from build123d import *

# Parameters (mm, degrees)
SKETCH1_W           = 94
SKETCH1_H           = 94
BOSS_EXTRUDE1_DEPTH = 11.3
SKETCH2_R           = 1.9
BOSS_EXTRUDE2_DEPTH = 2
SKETCH3_R           = 2.4
BOSS_EXTRUDE3_DEPTH = 17.9
SKETCH4_W           = 4
SKETCH4_H           = 7
CUT_EXTRUDE1_DEPTH  = 7.4


with BuildPart() as part:
    # Sketch1 → Boss-Extrude1 (new body)
    with BuildSketch(Plane(origin=(0, 0, 0), x_dir=(1, 0, 0), z_dir=(0, 1, 0))):
        with Locations((47, 47)):
            Rectangle(SKETCH1_W, SKETCH1_H)
    extrude(amount=BOSS_EXTRUDE1_DEPTH)

    # Sketch2 → Boss-Extrude2 (add)
    with BuildSketch(Plane.XZ):
        with Locations(Location((6.4, -6.4, 0), (0, 0, 270))):
            Circle(SKETCH2_R)
        with Locations(Location((6.4, -87.6, 0), (0, 0, 90))):
            Circle(SKETCH2_R)
        with Locations(Location((87.6, -87.6, 0), (0, 0, 270))):
            Circle(SKETCH2_R)
        with Locations(Location((87.6, -6.4, 0), (0, 0, 90))):
            Circle(SKETCH2_R)
    extrude(amount=BOSS_EXTRUDE2_DEPTH)

    # Sketch3 → Boss-Extrude3 (add)
    with BuildSketch(Plane(origin=(0, 11.3, 0), x_dir=(1, 0, 0), z_dir=(0, 1, 0))):
        with Locations(Location((47, 47, 0), (0, 0, 90))):
            Circle(SKETCH3_R)
    extrude(amount=BOSS_EXTRUDE3_DEPTH)

    # Sketch4 → Cut-Extrude1 (cut)
    with BuildSketch(Plane(origin=(0, 29.2, 0), x_dir=(1, 0, 0), z_dir=(0, 1, 0))):
        with Locations((45, 45.9)):
            Rectangle(SKETCH4_W, SKETCH4_H)
    extrude(amount=-CUT_EXTRUDE1_DEPTH, mode=Mode.SUBTRACT)


solid = part.part
Work out the finished part from the listing and answer in its coordinate system (mm). A direction names the side the tool comes from. Round coordinates to 2 decimals unless told otherwise and drop trailing zeros. Write each loop counter-clockwise with the first axis right and the second up, starting at its lowest first coordinate (ties: lowest second). Pieces come first, ordered by that corner, then holes. Notation, with made-up numbers: (-6, -32) -> (37, -32) arc R26 ccw to (37, 2) -> close; hole circle Ø6 at (-36.75, -36.75). An arc over 180 degrees is marked (long way). Answer as CSV lines item,"result". Start each with the question number.
(1) The part is cut by section D-D, the plane z = -6.4. Give the vertices of the cut face in (x, y), then the cut area to 3 significant figures.
(2) The part is cut by section B-B, the plane z = -47. Give the vertices of the cut face in (x, y).
(3) A tool of negligible diameter and unlimited length cuts with its end or side. For faces 1 (the flat face through (46, 6, -94)), 2 (the flat face through (46, 0, -48)), 3 (the flat face through (46, 21.8, -47)), from which of +Z, -Z, +X, -X, +Y, -Y can it reach the whole face along a straight path? Write none if from no direction.
(4) The mould has two halves that part along X. Classify faces 4 (the cylindrical face through (88.171, -0.986, -89.412)), 5 (the cylindrical face through (49.343, 18.136, -46.48)), 6 (the cylindrical face through (5.672, -0.986, -8.155)), 7 (the flat face through (6, -2, -88)): +X half, -X half, draft (parallel to the pull), parting line (faces both ways), or undercut.
(5) Each of these flat-tipped pins is pushed along its axis until it touches: pin 1 (1 mm diameter, centred on x = 38, z = -34.5, fed in from -Y); pin 2 (4 mm diameter, centred on y = 25.5, z = -47, fed in from -X); pin 3 (1.9 mm diameter, centred on x = 46, z = -47, fed in from +Y); pin 4 (5 mm diameter, centred on y = 19, z = -54, fed in from +X). Where does it stop, or does it pass through?
(6) The part is cut by section C-C, the plane y = 15.5. Give the vertices of the cut face in (x, z), then the cut area to 3 significant figures.
(7) Find the intervals of material crossed by probe 1 along Y at (x, z) = (67, -49); probe 2 along X at (y, z) = (25, -46.5), in increasing order.
(8) The part is cut by section A-A, the plane x = 6.4. Give the vertices of the cut face in (y, z).
Output values:
1,outline,"(0, 0) -> (4.5, 0) -> (4.5, -2) -> (8.3, -2) -> (8.3, 0) -> (85.7, 0) -> (85.7, -2) -> (89.5, -2) -> (89.5, 0) -> (94, 0) -> (94, 11.3) -> (0, 11.3) -> close"
1,area,"1,080 mm²"
2,outline,"(0, 0) -> (94, 0) -> (94, 11.3) -> (49.4, 11.3) -> (49.4, 29.2) -> (47, 29.2) -> (47, 21.8) -> (44.6, 21.8) -> (44.6, 11.3) -> (0, 11.3) -> close"
3,face 1,"-Z, +X, -X, +Y, -Y"
3,face 2,"-Y"
3,face 3,"+Z, -Z, -X, +Y"
4,face 4,"undercut"
4,face 5,"parting line"
4,face 6,"undercut"
4,face 7,"draft"
5,pin 1,"stops at y = 0"
5,pin 2,"stops at x = 47"
5,pin 3,"stops at y = 21.8"
5,pin 4,"passes through"
6,outline,"circle Ø4.8 at (47, -47)"
6,area,"18.1 mm²"
7,probe 1,"y = 0 to 11.3"
7,probe 2,"x = 47 to 49.35"
8,outline,"(-2, -89.5) -> (0, -89.5) -> (0, -94) -> (11.3, -94) -> (11.3, 0) -> (0, 0) -> (0, -4.5) -> (-2, -4.5) -> (-2, -8.3) -> (0, -8.3) -> (0, -85.7) -> (-2, -85.7) -> close"
